```python
from build123d import *

# Parameters (mm, degrees)
F2_R            = 2.5
F3_DEPTH        = 25.001
F2_R_2          = 1.5
F4_DEPTH        = 25.001
F4_COPIES_COUNT = 4


# Not quite as in the source:
# - a pattern or mirror of a feature is missing from the dataset's text; its kind, count and spacing are read off the source's solid


with BuildPart() as f1:
    # F0 (on Front) → F1 (revolve)
    with BuildSketch(Plane.XZ):
        with BuildLine():
            Line((0, 25), (0, 23.5))
            Line((0, 23.5), (20.5, 23.5))
            ThreePointArc((20.5, 23.5), (22.267766953, 22.767766953), (23, 21))
            Line((23, 21), (23, 0))
            Line((23, 0), (25, 0))
            Line((25, 0), (25, 14.5))
            Line((25, 14.5), (26, 14.5))
            Line((26, 14.5), (26, 15.5))
            Line((26, 15.5), (25, 15.5))
            Line((25, 15.5), (25, 21))
            ThreePointArc((25, 21), (23.8284271247, 23.8284271247), (21, 25))
            Line((21, 25), (0, 25))
        make_face()
    revolve(axis=Axis((24, 0, 0), (-1, 0, 0)))

    # F2 (on face) → F3 (cut, through all)
    with BuildSketch(Plane.YZ.offset(25)):
        Circle(F2_R)
    extrude(amount=-F3_DEPTH, mode=Mode.SUBTRACT)

    # F2 (on face) → F4 (cut, through all)
    with BuildSketch(Plane.YZ.offset(25)):
        with Locations((-12.7279220614, 12.7279220614)):
            Circle(F2_R_2)
    f4 = extrude(amount=-F4_DEPTH, mode=Mode.SUBTRACT)

    # F4_copies: F4 ×4 about axis
    f4_copies_axis = Axis((0, 0, 0), (1, 0, 0))
    for i in range(1, F4_COPIES_COUNT):
        add(f4.rotate(f4_copies_axis, i * 360 / F4_COPIES_COUNT), mode=Mode.SUBTRACT)


solid = f1.part
```
The model under review builds one solid part; all positions refer to its coordinate system, in mm. A direction names the side the tool comes from. Round coordinates to 2 decimals unless told otherwise and drop trailing zeros. Write each loop counter-clockwise with the first axis right and the second up, starting at its lowest first coordinate (ties: lowest second). Pieces come first, ordered by that corner, then holes. Notation, with made-up numbers: (77.25, 20.5) - (109.25, 20.5) arc R21 ccw to (109.25, 34.5) - close; hole circle Ø3 at (31.5, -39). An arc over 180 degrees is marked (long way). Answer as CSV lines item,"result". Start each with the question number.
(1) For faces 1 (the flat face through (25, 0, -3)), 2 (the cylindrical face through (10.4, 7.1, 22.4)), 3 (the cylindrical face through (24.014, -12.794, -14.226)), list the 3-axis set-ups (+Z, -Z, +X, -X, +Y, -Y) from which the entire face can be reached by the end or side of a thin tool; tool diameter is ignored.
(2) We need section C-C on x = 18.5. State the section outline as (y, z) points, plus the area to 3 significant figures.
(3) To check wall thickness, follow line 1 (Y direction, x = 11.75, z = 0); line 2 (Z direction, x = 2.5, y = -0.5) (3 decimals); line 3 (X direction, y = -3, z = -2). State the ranges of each line that lie inside material, in increasing order.
(4) We need section A-A on z = 0. State the section outline as (x, y) points.
(5) Draft analysis for pull direction Y (two halves, no side actions). For faces 4 (the flat face through (0, -17, -17)), 5 (the cylindrical face through (25.507, -12.864, 6.691)), 6 (the cylindrical face through (10.353, 7.509, 23.846)), 7 (the cylindrical face through (24.01, -0.54, -2.44)), state which applies: pulls with the +Y half, pulls with the -Y half, needs draft (parallel to the pull), parting line crosses it, or undercut.
(6) For pin 1 Ø2.5 at (y, z) = (-12.73, -12.73) entering from +X; pin 2 Ø3 at (y, z) = (-13.5, 19.5) entering from +X; pin 3 Ø6 at (y, z) = (10.5, 3) entering from -X; pin 4 Ø6 at (y, z) = (15, -13) entering from -X, all flat-tipped, find the tip position at first contact; note any pin that passes through.
Worked answers:
1,face 1,"+X"
1,face 2,"-X"
1,face 3,"+X, -X"
2,outline,"circle Ø50 at (0, 0); hole circle Ø47 at (0, 0)"
2,area,"229 mm²"
3,line 1,"-25 to -23.5, 23.5 to 25"
3,line 2,"-24.995 to -23.495, 23.495 to 24.995"
3,line 3,"23 to 25"
4,outline,"(0, -25) - (21, -25) arc R4 ccw to (25, -21) - (25, -15.5) - (26, -15.5) - (26, -14.5) - (25, -14.5) - (25, -2.5) - (23, -2.5) - (23, -21) arc R2.5 cw to (20.5, -23.5) - (0, -23.5) - close; (0, 23.5) - (20.5, 23.5) arc R2.5 cw to (23, 21) - (23, 2.5) - (25, 2.5) - (25, 14.5) - (26, 14.5) - (26, 15.5) - (25, 15.5) - (25, 21) arc R4 ccw to (21, 25) - (0, 25) - close"
5,face 4,"needs draft"
5,face 5,"undercut"
5,face 6,"parting line crosses it"
5,face 7,"undercut"
6,pin 1,"through"
6,pin 2,"x = 24.81"
6,pin 3,"x = 23"
6,pin 4,"x = 22.18"
